from build123d import *

# Parameters (mm, degrees)
EXTRUIR_L_MINA1_DEPTH   = 332.5
SALIENTE_EXTRUIR1_DEPTH = 0.5
SALIENTE_EXTRUIR2_START = -0.5
SALIENTE_EXTRUIR2_DEPTH = 0.5


with BuildPart() as part:
    # Croquis2 → Extruir-Lámina1 (new body)
    with BuildSketch(Plane(origin=(0, 0, 0), x_dir=(0, 0, -1), z_dir=(1, 0, 0))):
        with BuildLine():
            ThreePointArc((-64.178417971, 0), (-27.928417971, 19.344325839), (8.321582029, 0))
            Line((8.321582029, 0), (7.075512909, -0.835051942))
            ThreePointArc((7.075512909, -0.835051942), (-27.928417971, 17.844325839), (-62.93234885, -0.835051942))
            Line((-62.93234885, -0.835051942), (-64.178417971, 0))
        make_face()
    extrude(amount=EXTRUIR_L_MINA1_DEPTH)

    # Croquis3 → Saliente-Extruir1 (add)
    with BuildSketch(Plane.ZY):
        with BuildLine():
            Line((-7.075512909, -0.835051942), (62.93234885, -0.835051942))
            ThreePointArc((62.93234885, -0.835051942), (27.928417971, 17.844325839), (-7.075512909, -0.835051942))
        make_face()
    extrude(amount=-SALIENTE_EXTRUIR1_DEPTH)

    # Croquis4 → Saliente-Extruir2 (add)
    with BuildSketch(Plane(origin=(332.5, 0, 0), x_dir=(0, 0, -1), z_dir=(1, 0, 0)).offset(SALIENTE_EXTRUIR2_START)):
        with BuildLine():
            Line((-62.93234885, -0.835051942), (7.075512909, -0.835051942))
            ThreePointArc((7.075512909, -0.835051942), (-27.928417971, 17.844325839), (-62.93234885, -0.835051942))
        make_face()
    extrude(amount=SALIENTE_EXTRUIR2_DEPTH)


solid = part.part
The listing builds one solid part. Answer for the finished solid, in the listing's coordinates (mm). A direction names the side the tool comes from. Round coordinates to 2 decimals unless told otherwise and drop trailing zeros. Order: outer loops, then holes, each group sorted by start corner. A loop starts at its lowest first (then second) coordinate and runs counter-clockwise, first axis right, second up. Notation, with made-up numbers: (16.5, 36.25) - (67.5, 36.25) arc R11 cw to (67.5, 55.25) - close; hole circle Ø11 at (75.5, -26). An arc over 180 degrees is marked (long way). Write item = value, one per line. Start each with the question number.
1) Section A-A, the plane y = 9.75 is taken. Write down the section's boundary in (x, z), plus the area to 3 significant figures.
2) Section C-C, the plane x = 62.5 is taken. Write down the section's boundary in (y, z).
3) Section B-B, the plane z = 15.5 is taken. Write down the section's boundary in (x, y).
4) Straight lines are drawn through the part: L1, parallel to X at y = 9.5, z = 26; L2, parallel to Z at x = 27, y = 1.75; L3, parallel to Z at x = 124, y = 6. For each, find the intervals that lie inside material, in ascending order.
5) Section D-D, the plane z = 30 is taken. Write down the section's boundary in (x, y), plus the area to 3 significant figures.
6) Given pin 1 (2 mm diameter, centred on x = 215.5, z = 4, fed in from +Y); pin 2 (10 mm diameter, centred on x = 195.5, y = 15, fed in from +Z); pin 3 (8 mm diameter, centred on x = 283, y = 10, fed in from -Z), each flat-ended and moving along its own axis, determine where each tip first touches the part or whether it passes through.
7) For faces 4 (the cylindrical face through (163.93, 17.84, 27.35)), 5 (the flat face through (0, 7, 27)), determine the directions among +Z, -Z, +X, -X, +Y, -Y from which every point of the face is accessible in a straight line to the end or side of a thin tool.
8) For a pull along Z with two mould halves and no side action, classify faces 1 (the flat face through (332.5, 7, 28)), 2 (the cylindrical face through (163.92, 19.34, 28.53)), 3 (the flat face through (0.5, 7, 27)) as released by +Z, released by -Z, zero draft, split by the parting line, or undercut.
Results list:
q1.outline = (0, 0.63) - (332.5, 0.63) - (332.5, 55.23) - (0, 55.23) - close; hole (0.5, 3.1) - (332, 3.1) - (332, 52.76) - (0.5, 52.76) - close
q1.area = 1,690 mm^2
q2.outline = (-0.84, -7.08) - (0, -8.32) arc R43.64 ccw to (0, 64.18) - (-0.84, 62.93) arc R42.14 cw to start
q3.outline = (0, -0.84) - (0.5, -0.84) - (0.5, 15.97) - (332, 15.97) - (332, -0.84) - (332.5, -0.84) - (332.5, 17.54) - (0, 17.54) - close
q4.L1 = 0 to 0.5, 332 to 332.5
q4.L2 = -7.09 to -5.2, 61.05 to 62.94
q4.L3 = -3.48 to -1.36, 57.22 to 59.34
q5.outline = (0, -0.84) - (0.5, -0.84) - (0.5, 17.79) - (332, 17.79) - (332, -0.84) - (332.5, -0.84) - (332.5, 19.3) - (0, 19.3) - close
q5.area = 518 mm^2
q6.pin_1 = 12.84
q6.pin_2 = 54.91
q6.pin_3 = -3.48
q7.face_4 = -Y
q7.face_5 = +Z, -Z, -X, +Y, -Y
q8.face_1 = zero draft
q8.face_2 = split by the parting line
q8.face_3 = undercut
